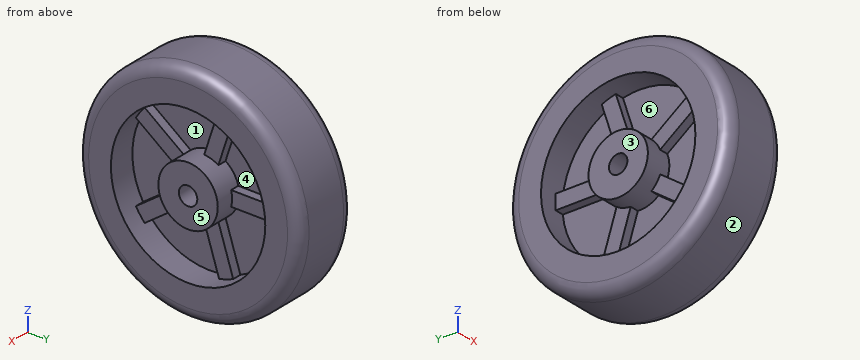
```python
from build123d import *

# Parameters (mm, degrees)
SKETCH_1_R               = 60
EXTRUDE_1_DEPTH          = 22.5
SKETCH_2_R               = 75
SKETCH_2_R_2             = 60
EXTRUDE_2_DEPTH          = 45
FILLET_1_R               = 8
SKETCH_3_R               = 52
SKETCH_3_R_2             = 20
CUT_EXTRUDE_1_DEPTH      = 18
SKETCH_4_R               = 6.2
CUT_EXTRUDE_2_DEPTH      = 116.217186348
EXTRUDE_START            = 6
EXTRUDE_3_DEPTH          = 6
PATTERN_CIRCULAR_1_COUNT = 5
MIRROR_START             = 6
MIRROR_2_COPY_1_DEPTH    = 6
MIRROR_2_COPY_2_DEPTH    = 6
MIRROR_2_COPY_3_DEPTH    = 6
MIRROR_2_COPY_4_DEPTH    = 6


with BuildPart() as part:
    # Sketch 1 → Extrude 1 (new, symmetric)
    with BuildSketch(Plane(origin=(0, 0, 0), x_dir=(0, 0, -1), z_dir=(1, 0, 0))):
        with Locations(Location((0, 0, 0), (0, 0, 180))):
            Circle(SKETCH_1_R)
    extrude(amount=EXTRUDE_1_DEPTH, both=True)

    # Sketch 3 → Cut-Extrude 1 (cut)
    with BuildSketch(Plane.ZY.offset(22.5)):
        Circle(SKETCH_3_R)
        Circle(SKETCH_3_R_2, mode=Mode.SUBTRACT)
    cut_extrude_1 = extrude(amount=-CUT_EXTRUDE_1_DEPTH, mode=Mode.SUBTRACT)

    # Sketch 4 → Cut-Extrude 2 (cut, through all)
    with BuildSketch(Plane.ZY.offset(22.5)):
        Circle(SKETCH_4_R)
    extrude(amount=-CUT_EXTRUDE_2_DEPTH, mode=Mode.SUBTRACT)


with BuildPart() as body_2:
    # Sketch 2 → Extrude 2 (new body)
    with BuildSketch(Plane(origin=(22.5, 0, 0), x_dir=(0, 0, -1), z_dir=(1, 0, 0))):
        Circle(SKETCH_2_R)
        Circle(SKETCH_2_R_2, mode=Mode.SUBTRACT)
    extrude(amount=-EXTRUDE_2_DEPTH)

    # Fillet 1
    fillet_1_edges = [body_2.edges().sort_by_distance(p)[0] for p in [
        (22.5, 0, 75),
        (-22.5, 0, 75),
    ]]
    fillet(fillet_1_edges, radius=FILLET_1_R)


    add(part.part)  # Extrude 3 merges part
    # Sketch 5 → Extrude 3 (add)
    with BuildSketch(Plane.ZY.offset(4.5).offset(EXTRUDE_START)):
        with BuildLine():
            ThreePointArc((5, 51.759057178), (0, 52), (-5, 51.759057178))
            Line((-5, 51.759057178), (-5, 19.364916731))
            ThreePointArc((-5, 19.364916731), (0, 20), (5, 19.364916731))
            Line((5, 19.364916731), (5, 51.759057178))
        make_face()
    extrude_3 = extrude(amount=-EXTRUDE_3_DEPTH)

    # Pattern Circular 1: Extrude 3 ×5 about axis
    pattern_circular_1_axis = Axis((0, 0, 0), (1, 0, 0))
    for i in range(1, PATTERN_CIRCULAR_1_COUNT):
        add(extrude_3.rotate(pattern_circular_1_axis, i * 360 / PATTERN_CIRCULAR_1_COUNT))

    # Mirror 2: Cut-Extrude 1, Extrude 3 across plane
    add(cut_extrude_1.mirror(Plane(origin=(0, 0, 0), x_dir=(0, 0, 1), z_dir=(1, 0, 0))), mode=Mode.SUBTRACT)
    add(extrude_3.mirror(Plane(origin=(0, 0, 0), x_dir=(0, 0, 1), z_dir=(1, 0, 0))))

    # Mirror 2 copy 1 sketch → Mirror 2 copy 1 (add)
    with BuildSketch(Plane(origin=(4.5, 0, 0), x_dir=(0, -0.9510565162951535, 0.30901699437494745), z_dir=(1, 0, 0)).offset(MIRROR_START)):
        with BuildLine():
            ThreePointArc((5, -51.759057178), (0, -52), (-5, -51.759057178))
            Line((-5, -51.759057178), (-5, -19.364916731))
            ThreePointArc((-5, -19.364916731), (0, -20), (5, -19.364916731))
            Line((5, -19.364916731), (5, -51.759057178))
        make_face()
    extrude(amount=-MIRROR_2_COPY_1_DEPTH)

    # Mirror 2 copy 2 sketch → Mirror 2 copy 2 (add)
    with BuildSketch(Plane(origin=(4.5, 0, 0), x_dir=(0, -0.5877852522924732, -0.8090169943749473), z_dir=(1, 0, 0)).offset(MIRROR_START)):
        with BuildLine():
            ThreePointArc((5, -51.759057178), (0, -52), (-5, -51.759057178))
            Line((-5, -51.759057178), (-5, -19.364916731))
            ThreePointArc((-5, -19.364916731), (0, -20), (5, -19.364916731))
            Line((5, -19.364916731), (5, -51.759057178))
        make_face()
    extrude(amount=-MIRROR_2_COPY_2_DEPTH)

    # Mirror 2 copy 3 sketch → Mirror 2 copy 3 (add)
    with BuildSketch(Plane(origin=(4.5, 0, 0), x_dir=(0, 0.587785252292473, -0.8090169943749476), z_dir=(1, 0, 0)).offset(MIRROR_START)):
        with BuildLine():
            ThreePointArc((5, -51.759057178), (0, -52), (-5, -51.759057178))
            Line((-5, -51.759057178), (-5, -19.364916731))
            ThreePointArc((-5, -19.364916731), (0, -20), (5, -19.364916731))
            Line((5, -19.364916731), (5, -51.759057178))
        make_face()
    extrude(amount=-MIRROR_2_COPY_3_DEPTH)

    # Mirror 2 copy 4 sketch → Mirror 2 copy 4 (add)
    with BuildSketch(Plane(origin=(4.5, 0, 0), x_dir=(0, 0.9510565162951536, 0.30901699437494723), z_dir=(1, 0, 0)).offset(MIRROR_START)):
        with BuildLine():
            ThreePointArc((5, -51.759057178), (0, -52), (-5, -51.759057178))
            Line((-5, -51.759057178), (-5, -19.364916731))
            ThreePointArc((-5, -19.364916731), (0, -20), (5, -19.364916731))
            Line((5, -19.364916731), (5, -51.759057178))
        make_face()
    extrude(amount=-MIRROR_2_COPY_4_DEPTH)


solid = body_2.part
```
For this review, take the finished solid that the model builds, in its own axes (mm). Face numbers are marked on the shaded views. A direction names the side the tool comes from. Round coordinates to 2 decimals unless told otherwise and drop trailing zeros. Loops run counter-clockwise (first coordinate to the right, second up) from the corner with the lowest first, then second, coordinate; pieces in that order, holes last.
Q1. Mouldability with a two-part tool opening along Z and no side actions: class the marked faces 1, 2 and 3 as +Z half, -Z half, draft (parallel to the pull), parting line (faces both ways), or undercut.
Result sheet:
face 1: undercut
face 2: parting line
face 3: draft
Q2. Add section A-A on z = 0. Write out the cut boundary in (x, y), plus the area to 3 significant figures.
Result sheet:
outline: (-22.5, -67) arc R8 ccw to (-14.5, -75) - (14.5, -75) arc R8 ccw to (22.5, -67) - (22.5, -52) - (4.5, -52) - (4.5, -20) - (22.5, -20) - (22.5, -6.2) - (-22.5, -6.2) - (-22.5, -20) - (-4.5, -20) - (-4.5, -52) - (-22.5, -52) - close; (-22.5, 6.2) - (22.5, 6.2) - (22.5, 20) - (10.5, 20) - (10.5, 52) - (22.5, 52) - (22.5, 67) arc R8 ccw to (14.5, 75) - (-14.5, 75) arc R8 ccw to (-22.5, 67) - (-22.5, 52) - (-10.5, 52) - (-10.5, 20) - (-22.5, 20) - close
area: 4,220 mm2
Q3. Insertion check: pin 1 Ø6 at (y, z) = (7.5, -26.5) entering from -X; pin 2 Ø8 at (x, y) = (2.5, 59.5) entering from +Z; pin 3 Ø2 at (x, y) = (-16.5, -55.5) entering from +Z. Each pin has a flat end and moves straight along its axis. Give the tip position at first contact, or say it passes through.
Result sheet:
pin 1: stops at x = -10.5
pin 2: stops at z = 50.45
pin 3: stops at z = 51.21
Q4. To check wall thickness, follow line 1 along Y through (x, z) = (11.5, 0); line 2 along Z through (x, y) = (5, -0.5); line 3 along Y through (x, z) = (6, -40.5). State the ranges of each line that lie inside material, in increasing order.
Result sheet:
line 1: y = -75 to -52, -20 to -6.2, 6.2 to 20, 52 to 75
line 2: z = -75 to -52, -19.99 to -6.18, 6.18 to 19.99, 52 to 75
line 3: y = -63.12 to -32.62, 7.9 to 18.42, 32.62 to 63.12
Q5. Add section B-B on x = 0. Write out the cut boundary in (y, z), plus the area to 3 significant figures.
Result sheet:
outline: circle Ø150 at (0, 0); hole circle Ø12.4 at (0, 0)
area: 17,600 mm2
Q6. Machinability: for the marked faces 4, 5 and 6, which of the approach directions +Z, -Z, +X, -X, +Y, -Y give a long, thin tool a straight path to every point of the face, cutting with its end or side? Answer none if there is none.
Result sheet:
face 4: +X
face 5: +Z, -Z, +X, +Y, -Y
face 6: -X
